from build123d import *

# Parameters (mm, degrees)
F0_R     = 2.175
F0_R_2   = 4.4
F0_R_3   = 5.15
F1_DEPTH = 6.1
F2_R     = 2.1
F3_DEPTH = 6.101


with BuildPart() as f1:
    # F0 (on Front) → F1 (new body)
    with BuildSketch(Plane.XZ):
        with BuildLine():
            ThreePointArc((-28.172905, 14.582949), (-32.408847, 14.865425), (-35.335057, 11.789667))
            ThreePointArc((-35.335057, 11.789667), (-37.25, 0), (-35.335057, -11.789667))
            ThreePointArc((-35.335057, -11.789667), (-32.408847, -14.865425), (-28.172905, -14.582949))
            ThreePointArc((-28.172905, -14.582949), (-16.263456, -16.263456), (-14.582949, -28.172905))
            ThreePointArc((-14.582949, -28.172905), (-14.865425, -32.408847), (-11.789667, -35.335057))
            ThreePointArc((-11.789667, -35.335057), (0, -37.25), (11.789667, -35.335057))
            ThreePointArc((11.789667, -35.335057), (14.865425, -32.408847), (14.582949, -28.172905))
            ThreePointArc((14.582949, -28.172905), (16.263456, -16.263456), (28.172905, -14.582949))
            ThreePointArc((28.172905, -14.582949), (32.408847, -14.865425), (35.335057, -11.789667))
            ThreePointArc((35.335057, -11.789667), (37.25, 0), (35.335057, 11.789667))
            ThreePointArc((35.335057, 11.789667), (32.408847, 14.865425), (28.172905, 14.582949))
            ThreePointArc((28.172905, 14.582949), (16.263456, 16.263456), (14.582949, 28.172905))
            ThreePointArc((14.582949, 28.172905), (14.865425, 32.408847), (11.789667, 35.335057))
            ThreePointArc((11.789667, 35.335057), (0, 37.25), (-11.789667, 35.335057))
            ThreePointArc((-11.789667, 35.335057), (-14.865425, 32.408847), (-14.582949, 28.172905))
            ThreePointArc((-14.582949, 28.172905), (-16.263456, 16.263456), (-28.172905, 14.582949))
        make_face()
        with Locations((0, -28.8)):
            Circle(F0_R, mode=Mode.SUBTRACT)
        with Locations((0, -17.85)):
            Circle(F0_R_2, mode=Mode.SUBTRACT)
        with Locations((-28.8, 0)):
            Circle(F0_R, mode=Mode.SUBTRACT)
        with Locations((-17.85, 0)):
            Circle(F0_R_2, mode=Mode.SUBTRACT)
        Circle(F0_R_3, mode=Mode.SUBTRACT)
        with Locations((0, 17.85)):
            Circle(F0_R_2, mode=Mode.SUBTRACT)
        with Locations((0, 28.8)):
            Circle(F0_R, mode=Mode.SUBTRACT)
        with Locations((17.85, 0)):
            Circle(F0_R_2, mode=Mode.SUBTRACT)
        with Locations((28.8, 0)):
            Circle(F0_R, mode=Mode.SUBTRACT)
    extrude(amount=F1_DEPTH)

    # F2 (on face) → F3 (cut, through all)
    with BuildSketch(Plane.XZ.offset(6.1)):
        with Locations((-10.606602, 10.606602)):
            Circle(F2_R)
        with Locations((-10.606602, -10.606602)):
            Circle(F2_R)
        with Locations((10.606602, -10.606602)):
            Circle(F2_R)
        with Locations((10.606602, 10.606602)):
            Circle(F2_R)
    extrude(amount=-F3_DEPTH, mode=Mode.SUBTRACT)


solid = f1.part
Geometry: final body of the model. Coordinates: model frame, mm. Coordinates: 2 decimals unless noted, no trailing zeros. Loops run counter-clockwise (first coordinate to the right, second up) from the corner with the lowest first, then second, coordinate; pieces in that order, holes last. Notation, with made-up numbers: M 29.5,-39.75 L 84.5,-39.75 A28 cw 84.5,-0.75 Z; hole C 88.5,89.5 d6. An arc over 180 degrees is marked long. One line per item, written item: value. Start each with the question number.
1) Pin query (flat end, axial travel): P1, Ø2, axis at y = -2.5, z = 23.5, coming from the -X side; P2, Ø3, axis at x = 22.5, y = -1.5, coming from the +Z side; P3, Ø3, axis at y = -1, z = 27, coming from the -X side. Return the tip coordinate at first contact, or that it passes through.
2) Material intervals for L1, parallel to Z at x = -17.5, y = -3.25; L2, parallel to X at y = -4.5, z = 9, sorted ascending. Write a range as from..to.
3) Draft query along Z for faces 1 (the cylindrical face through (-32.35, -3.01, 14.89)), 2 (the cylindrical face through (27.197, -3.007, 1.47)), 3 (the cylindrical face through (-8.604, -3.093, -9.976)), 4 (the cylindrical face through (-32.47, -3.01, -14.84)). Return one class per face: released by +Z, released by -Z, zero draft, split by the parting line, or undercut.
4) Cut plane D-D (z = 19.5). Return loops of the section in (x, y).
5) Cut plane C-C (y = -2). Count the separate pieces of the cut face and the enclosed holes in it, then the cut area to 3 significant figures.
6) Cut plane A-A (z = 0). Return loops of the section in (x, y) (3 decimals), then the cut area to 3 significant figures.
7) Cut plane B-B (x = 17.85). Return loops of the section in (y, z).
Evaluation:
1. P1: x = -13.4
1. P2: z = 13.61
1. P3: x = -14.75
2. L1: -15.21..-4.39, 4.39..15.21
2. L2: -36.15..-11.96, -9.25..9.25, 11.96..36.15
3. face 1: released by +Z
3. face 2: undercut
3. face 3: undercut
3. face 4: released by -Z
4. outline: M -14.1,-6.1 L -4.08,-6.1 L -4.08,0 L -14.1,0 Z; M 4.08,-6.1 L 14.1,-6.1 L 14.1,0 L 4.08,0 Z
5. separate pieces: 1
5. enclosed holes: 13
5. area: 2,910 mm^2
6. outline: M -37.25,-6.1 L -30.975,-6.1 L -30.975,0 L -37.25,0 Z; M -26.625,-6.1 L -22.25,-6.1 L -22.25,0 L -26.625,0 Z; M -13.45,-6.1 L -5.15,-6.1 L -5.15,0 L -13.45,0 Z; M 5.15,-6.1 L 13.45,-6.1 L 13.45,0 L 5.15,0 Z; M 22.25,-6.1 L 26.625,-6.1 L 26.625,0 L 22.25,0 Z; M 30.975,-6.1 L 37.25,-6.1 L 37.25,0 L 30.975,0 Z
6. area: 231 mm^2
7. outline: M -6.1,-14.97 L 0,-14.97 L 0,-4.4 L -6.1,-4.4 Z; M -6.1,4.4 L 0,4.4 L 0,14.97 L -6.1,14.97 Z
